from build123d import *

# Parameters (mm, degrees)
F1_DEPTH = 63.5
F0_W     = 25.4
F0_H     = 14.2875
F2_DEPTH = 25.4
F3_DEPTH = 7.9375


with BuildPart() as f1:
    # F0 (on Front) → F1 (new body, symmetric)
    with BuildSketch(Plane.XZ):
        Polygon((41.275, -9.525), (41.275, 9.525), (26.524457, 9.525), (-41.275, 9.525), (-41.275, -9.525), align=None)
    extrude(amount=F1_DEPTH, both=True)

    # F0 (on Front) → F2 (join, symmetric)
    with BuildSketch(Plane.XZ):
        with BuildLine():
            Line((26.524457, 9.525), (41.275, 9.525))
            Line((41.275, 9.525), (41.275, 46.0502))
            ThreePointArc((41.275, 46.0502), (45.92468, 57.27552), (57.15, 61.9252))
            Line((57.15, 61.9252), (76.2, 61.9252))
            Line((76.2, 61.9252), (76.2, 76.2127))
            Line((76.2, 76.2127), (101.6, 76.2127))
            Line((101.6, 76.2127), (101.6, 76.675743))
            Line((101.6, 76.675743), (57.15, 76.675743))
            ThreePointArc((57.15, 76.675743), (35.494471, 67.705729), (26.524457, 46.0502))
            Line((26.524457, 46.0502), (26.524457, 9.525))
        make_face()
        with Locations((88.9, 69.06895)):
            Rectangle(F0_W, F0_H)
    extrude(amount=F2_DEPTH, both=True)

    # F0 (on Front) → F3 (join, symmetric)
    with BuildSketch(Plane.XZ):
        with BuildLine():
            Line((-41.275, 9.525), (26.524457, 9.525))
            Line((26.524457, 9.525), (26.524457, 46.0502))
            ThreePointArc((26.524457, 46.0502), (35.494471, 67.705729), (57.15, 76.675743))
            add(Edge.make_bspline(
                [(-41.275, 9.525), (-28.42545, 44.060338), (-4.196861, 78.073546), (57.15, 76.675743)],
                knots=[0, 0, 0, 0, 119.149918, 119.149918, 119.149918, 119.149918], degree=3))
        make_face()
    extrude(amount=F3_DEPTH, both=True)

    # F0 (on Front) → F4 (revolve)
    with BuildSketch(Plane.XZ):
        Polygon((101.6, 76.2127), (101.6, 61.9252), (101.6, 47.6377), (127, 47.6377), (127, 76.2127), align=None)
    revolve(axis=Axis((101.6, 0, 62.156721), (0, 0, 1)))


solid = f1.part
CAD build for the part. Positions are in the model's coordinates, mm. A direction names the side the tool comes from. Coordinates: 2 decimals unless noted, no trailing zeros. Write each loop counter-clockwise with the first axis right and the second up, starting at its lowest first coordinate (ties: lowest second). Pieces come first, ordered by that corner, then holes. Notation, with made-up numbers: M 21,20 L 54,20 A34 cw 54,51 Z; hole C -12,32 d6. An arc over 180 degrees is marked long. Answer as a JSON object with one key per item and string values. Group by question number.
1) Saw through at A-A (y = -18). Write the cut outline in (x, z) (3 decimals), plus the area to 3 significant figures.
2) Pin check, flat tips, straight feed: pin 1 Ø8.5 at (y, z) = (-19, 23.5) entering from -X; pin 2 Ø12 at (x, y) = (48.5, 31) entering from +Z; pin 3 Ø5 at (x, y) = (60.5, 2.5) entering from +Z; pin 4 Ø20 at (x, z) = (61, 29) entering from -Y. Stop position of each tip, or through.
3) Saw through at B-B (x = 79). Write the cut outline in (y, z), plus the area to 3 significant figures.
4) Tool access for faces 4 (the face through (26.524, -17, 28)), 5 (the face through (45.8, -0.36, 57.15)), 6 (the face through (111, 0, 76.213)), 7 (the face through (-4, 7.938, 37)), 8 (the face through (46.9, 25.4, 58.5)): list every direction of +Z, -Z, +X, -X, +Y, -Y with a clear straight run to the whole face (end or side of a thin tool).
5) Mould opens along X. For faces 1 (the face through (35.73, -16.79, 67.94)), 2 (the face through (102, 0, 47.638)), 3 (the face through (69, 0, 61.925)) say: +X half, -X half, draft (parallel to the pull), parting line (faces both ways), or undercut.
6) Saw through at C-C (y = -50). Write the cut outline in (x, z) (3 decimals).
7) Wall check: line 1 (X direction, y = -19, z = -3.5) (3 decimals); line 2 (Z direction, x = 98.5, y = -22); line 3 (X direction, y = -20.5, z = 48). Give the ranges that are in metal, low to high. Write a range as from..to.
Values follow:
{
 "1": {"outline": "M -41.275,-9.525 L 41.275,-9.525 L 41.275,46.05 A15.875 cw 57.15,61.925 L 83.679,61.925 L 83.679,47.638 L 119.521,47.638 L 119.521,76.213 L 101.6,76.213 L 101.6,76.676 L 57.15,76.676 A30.626 ccw 26.524,46.05 L 26.524,9.525 L -41.275,9.525 Z", "area": "4,070 mm2"},
 "2": {"pin 1": "stops at x = 26.52", "pin 2": "stops at z = 75.98", "pin 3": "stops at z = 76.68", "pin 4": "passes through"},
 "3": {"outline": "M -25.4,61.93 L -11.59,61.93 L -11.59,47.64 L 11.59,47.64 L 11.59,61.93 L 25.4,61.93 L 25.4,76.68 L -25.4,76.68 Z", "area": "1,080 mm2"},
 "4": {"face 4": "+Z, -X, -Y", "face 5": "-Z, +Y, -Y", "face 6": "+Z, +X, +Y, -Y", "face 7": "+Z, -X, +Y", "face 8": "+Z, +X, -X, +Y"},
 "5": {"face 1": "-X half", "face 2": "draft", "face 3": "undercut"},
 "6": {"outline": "M -41.275,-9.525 L 41.275,-9.525 L 41.275,9.525 L -41.275,9.525 Z"},
 "7": {"line 1": "x = -41.275..41.275", "line 2": "z = 47.64..76.68", "line 3": "x = 26.59..41.4, 86.6..116.6"}
}
